Input: part model. Units: mm. Frame: model coordinates. Face numbers are marked on the shaded views. A direction names the side the tool comes from. Give positions to 0.01 mm unless a question says otherwise; leave off trailing zeros. Write each loop counter-clockwise with the first axis right and the second up, starting at its lowest first coordinate (ties: lowest second). Pieces come first, ordered by that corner, then holes. Notation, with made-up numbers: (77.25, -21.5) - (115.25, -21.5) arc R20 cw to (115.25, 1.5) - close; hole circle Ø8 at (5.25, 11). An arc over 180 degrees is marked (long way). Use a Markdown table: item, result. Add a question column.
1. Mould query, pull axis Y, two halves, no side actions, for the marked faces 1, 2, 3 and 4. Classes: released by +Y, released by -Y, zero draft, split by the parting line, or undercut.
2. Section query C-C, the plane z = -4. Return loops of the section in (x, y).
3. Pin query (flat end, axial travel): pin 1 (5 mm diameter, centred on x = -79, z = -7, fed in from +Y); pin 2 (4 mm diameter, centred on y = 70.5, z = -11.5, fed in from +X); pin 3 (5 mm diameter, centred on y = -74, z = -12.5, fed in from +X) (3 decimals); pin 4 (1.5 mm diameter, centred on x = -24.5, y = 76.5, fed in from +Z). Return the tip coordinate at first contact, or that it passes through.
4. Set-up query: the marked faces 5 and 6. Return all of +Z, -Z, +X, -X, +Y, -Y with unobstructed straight access to the full face (end or side cutting, diameter ignored); none if empty.
5. Section query B-B, the plane y = -5.5. Return loops of the section in (x, z) (3 decimals), plus the area to 3 significant figures.
6. Material intervals for probe 1 along Y at (x, z) = (50, 3.25); probe 2 along X at (y, z) = (-47.5, 0.25); probe 3 along Y at (x, z) = (-48.5, -2.5), sorted ascending.
7. Section query D-D, the plane y = 96. Return loops of the section in (x, z) (3 decimals).
```python
from build123d import *

# Parameters (mm, degrees)
F1_DEPTH = 15.875
F2_DEPTH = 9.525
F3_DEPTH = 6.35


with BuildPart() as f1:
    # F0 (on Top) → F1 (new body)
    with BuildSketch(Plane.XY):
        with BuildLine():
            ThreePointArc((-69.85, 109.5375), (-101.2808964237, 96.5183964237), (-114.3, 65.0875))
            Line((-114.3, 65.0875), (-114.3, -65.0875))
            ThreePointArc((-114.3, -65.0875), (-101.2808964237, -96.5183964237), (-69.85, -109.5375))
            Line((-69.85, -109.5375), (69.85, -109.5375))
            ThreePointArc((69.85, -109.5375), (101.2808964237, -96.5183964237), (114.3, -65.0875))
            Line((114.3, -65.0875), (114.3, 65.0875))
            ThreePointArc((114.3, 65.0875), (101.2808964237, 96.5183964237), (69.85, 109.5375))
            Line((69.85, 109.5375), (-69.85, 109.5375))
        make_face()
        with BuildLine():
            Line((-69.85, 103.187499407), (69.85, 103.187499407))
            ThreePointArc((69.85, 103.187499407), (96.7907679439, 92.0282679439), (107.949999407, 65.0875))
            Line((107.949999407, 65.0875), (107.949999407, -65.0875))
            ThreePointArc((107.949999407, -65.0875), (96.7907679439, -92.0282679439), (69.85, -103.187499407))
            Line((69.85, -103.187499407), (-69.85, -103.187499407))
            ThreePointArc((-69.85, -103.187499407), (-96.7907679439, -92.0282679439), (-107.949999407, -65.0875))
            Line((-107.949999407, -65.0875), (-107.949999407, 65.0875))
            ThreePointArc((-107.949999407, 65.0875), (-96.7907679439, 92.0282679439), (-69.85, 103.187499407))
        make_face(mode=Mode.SUBTRACT)
        with BuildLine():
            ThreePointArc((107.949999407, 65.0875), (96.7907679439, 92.0282679439), (69.85, 103.187499407))
            Line((69.85, 103.187499407), (-69.85, 103.187499407))
            ThreePointArc((-69.85, 103.187499407), (-96.7907679439, 92.0282679439), (-107.949999407, 65.0875))
            Line((-107.949999407, 65.0875), (-107.949999407, -65.0875))
            ThreePointArc((-107.949999407, -65.0875), (-96.7907679439, -92.0282679439), (-69.85, -103.187499407))
            Line((-69.85, -103.187499407), (69.85, -103.187499407))
            ThreePointArc((69.85, -103.187499407), (96.7907679439, -92.0282679439), (107.949999407, -65.0875))
            Line((107.949999407, -65.0875), (107.949999407, 65.0875))
        make_face()
        with BuildLine():
            Line((-107.187999407, -65.0875), (-107.187999407, 65.0875))
            ThreePointArc((-107.187999407, 65.0875), (-96.2519525766, 91.4894525766), (-69.85, 102.425499407))
            Line((-69.85, 102.425499407), (69.85, 102.425499407))
            ThreePointArc((69.85, 102.425499407), (96.2519525766, 91.4894525766), (107.187999407, 65.0875))
            Line((107.187999407, 65.0875), (107.187999407, -65.0875))
            ThreePointArc((107.187999407, -65.0875), (96.2519525766, -91.4894525766), (69.85, -102.425499407))
            Line((69.85, -102.425499407), (-69.85, -102.425499407))
            ThreePointArc((-69.85, -102.425499407), (-96.2519525766, -91.4894525766), (-107.187999407, -65.0875))
        make_face(mode=Mode.SUBTRACT)
        with BuildLine():
            ThreePointArc((-69.85, 102.425499407), (-96.2519525766, 91.4894525766), (-107.187999407, 65.0875))
            Line((-107.187999407, 65.0875), (-107.187999407, -65.0875))
            ThreePointArc((-107.187999407, -65.0875), (-96.2519525766, -91.4894525766), (-69.85, -102.425499407))
            Line((-69.85, -102.425499407), (69.85, -102.425499407))
            ThreePointArc((69.85, -102.425499407), (96.2519525766, -91.4894525766), (107.187999407, -65.0875))
            Line((107.187999407, -65.0875), (107.187999407, 65.0875))
            ThreePointArc((107.187999407, 65.0875), (96.2519525766, 91.4894525766), (69.85, 102.425499407))
            Line((69.85, 102.425499407), (-69.85, 102.425499407))
        make_face()
        with BuildLine():
            Line((-89.662, -65.0875), (-89.662, 65.0875))
            ThreePointArc((-89.662, 65.0875), (-83.8591995489, 79.0966995489), (-69.85, 84.8995))
            Line((-69.85, 84.8995), (69.85, 84.8995))
            ThreePointArc((69.85, 84.8995), (83.8591995489, 79.0966995489), (89.662, 65.0875))
            Line((89.662, 65.0875), (89.662, -65.0875))
            ThreePointArc((89.662, -65.0875), (83.8591995489, -79.0966995489), (69.85, -84.8995))
            Line((69.85, -84.8995), (-69.85, -84.8995))
            ThreePointArc((-69.85, -84.8995), (-83.8591995489, -79.0966995489), (-89.662, -65.0875))
        make_face(mode=Mode.SUBTRACT)
        with BuildLine():
            ThreePointArc((-69.85, 84.8995), (-83.8591995489, 79.0966995489), (-89.662, 65.0875))
            Line((-89.662, 65.0875), (-89.662, -65.0875))
            ThreePointArc((-89.662, -65.0875), (-83.8591995489, -79.0966995489), (-69.85, -84.8995))
            Line((-69.85, -84.8995), (69.85, -84.8995))
            ThreePointArc((69.85, -84.8995), (83.8591995489, -79.0966995489), (89.662, -65.0875))
            Line((89.662, -65.0875), (89.662, 65.0875))
            ThreePointArc((89.662, 65.0875), (83.8591995489, 79.0966995489), (69.85, 84.8995))
            Line((69.85, 84.8995), (-69.85, 84.8995))
        make_face()
        with BuildLine():
            ThreePointArc((-88.9, 65.0875), (-83.3203841816, 78.5578841816), (-69.85, 84.1375))
            Line((-69.85, 84.1375), (69.85, 84.1375))
            ThreePointArc((69.85, 84.1375), (83.3203841816, 78.5578841816), (88.9, 65.0875))
            Line((88.9, 65.0875), (88.9, -65.0875))
            ThreePointArc((88.9, -65.0875), (83.3203841816, -78.5578841816), (69.85, -84.1375))
            Line((69.85, -84.1375), (-69.85, -84.1375))
            ThreePointArc((-69.85, -84.1375), (-83.3203841816, -78.5578841816), (-88.9, -65.0875))
            Line((-88.9, -65.0875), (-88.9, 65.0875))
        make_face(mode=Mode.SUBTRACT)
        with BuildLine():
            Line((69.85, 84.1375), (-69.85, 84.1375))
            ThreePointArc((-69.85, 84.1375), (-83.3203841816, 78.5578841816), (-88.9, 65.0875))
            Line((-88.9, 65.0875), (-88.9, -65.0875))
            ThreePointArc((-88.9, -65.0875), (-83.3203841816, -78.5578841816), (-69.85, -84.1375))
            Line((-69.85, -84.1375), (69.85, -84.1375))
            ThreePointArc((69.85, -84.1375), (83.3203841816, -78.5578841816), (88.9, -65.0875))
            Line((88.9, -65.0875), (88.9, 65.0875))
            ThreePointArc((88.9, 65.0875), (83.3203841816, 78.5578841816), (69.85, 84.1375))
        make_face()
        with BuildLine():
            Line((-69.85, 77.7875), (69.85, 77.7875))
            ThreePointArc((69.85, 77.7875), (78.8302561211, 74.0677561211), (82.55, 65.0875))
            Line((82.55, 65.0875), (82.55, -65.0875))
            ThreePointArc((82.55, -65.0875), (78.8302561211, -74.0677561211), (69.85, -77.7875))
            Line((69.85, -77.7875), (-69.85, -77.7875))
            ThreePointArc((-69.85, -77.7875), (-78.8302561211, -74.0677561211), (-82.55, -65.0875))
            Line((-82.55, -65.0875), (-82.55, 65.0875))
            ThreePointArc((-82.55, 65.0875), (-78.8302561211, 74.0677561211), (-69.85, 77.7875))
        make_face(mode=Mode.SUBTRACT)
    extrude(amount=-F1_DEPTH)

    # F0 (on Top) → F2 (cut)
    with BuildSketch(Plane.XY):
        with BuildLine():
            ThreePointArc((107.949999407, 65.0875), (96.7907679439, 92.0282679439), (69.85, 103.187499407))
            Line((69.85, 103.187499407), (-69.85, 103.187499407))
            ThreePointArc((-69.85, 103.187499407), (-96.7907679439, 92.0282679439), (-107.949999407, 65.0875))
            Line((-107.949999407, 65.0875), (-107.949999407, -65.0875))
            ThreePointArc((-107.949999407, -65.0875), (-96.7907679439, -92.0282679439), (-69.85, -103.187499407))
            Line((-69.85, -103.187499407), (69.85, -103.187499407))
            ThreePointArc((69.85, -103.187499407), (96.7907679439, -92.0282679439), (107.949999407, -65.0875))
            Line((107.949999407, -65.0875), (107.949999407, 65.0875))
        make_face()
        with BuildLine():
            Line((-107.187999407, -65.0875), (-107.187999407, 65.0875))
            ThreePointArc((-107.187999407, 65.0875), (-96.2519525766, 91.4894525766), (-69.85, 102.425499407))
            Line((-69.85, 102.425499407), (69.85, 102.425499407))
            ThreePointArc((69.85, 102.425499407), (96.2519525766, 91.4894525766), (107.187999407, 65.0875))
            Line((107.187999407, 65.0875), (107.187999407, -65.0875))
            ThreePointArc((107.187999407, -65.0875), (96.2519525766, -91.4894525766), (69.85, -102.425499407))
            Line((69.85, -102.425499407), (-69.85, -102.425499407))
            ThreePointArc((-69.85, -102.425499407), (-96.2519525766, -91.4894525766), (-107.187999407, -65.0875))
        make_face(mode=Mode.SUBTRACT)
        with BuildLine():
            ThreePointArc((-69.85, 102.425499407), (-96.2519525766, 91.4894525766), (-107.187999407, 65.0875))
            Line((-107.187999407, 65.0875), (-107.187999407, -65.0875))
            ThreePointArc((-107.187999407, -65.0875), (-96.2519525766, -91.4894525766), (-69.85, -102.425499407))
            Line((-69.85, -102.425499407), (69.85, -102.425499407))
            ThreePointArc((69.85, -102.425499407), (96.2519525766, -91.4894525766), (107.187999407, -65.0875))
            Line((107.187999407, -65.0875), (107.187999407, 65.0875))
            ThreePointArc((107.187999407, 65.0875), (96.2519525766, 91.4894525766), (69.85, 102.425499407))
            Line((69.85, 102.425499407), (-69.85, 102.425499407))
        make_face()
        with BuildLine():
            Line((-89.662, -65.0875), (-89.662, 65.0875))
            ThreePointArc((-89.662, 65.0875), (-83.8591995489, 79.0966995489), (-69.85, 84.8995))
            Line((-69.85, 84.8995), (69.85, 84.8995))
            ThreePointArc((69.85, 84.8995), (83.8591995489, 79.0966995489), (89.662, 65.0875))
            Line((89.662, 65.0875), (89.662, -65.0875))
            ThreePointArc((89.662, -65.0875), (83.8591995489, -79.0966995489), (69.85, -84.8995))
            Line((69.85, -84.8995), (-69.85, -84.8995))
            ThreePointArc((-69.85, -84.8995), (-83.8591995489, -79.0966995489), (-89.662, -65.0875))
        make_face(mode=Mode.SUBTRACT)
    extrude(amount=F2_DEPTH, mode=Mode.SUBTRACT)

    # F0 (on Top) → F3 (join)
    with BuildSketch(Plane.XY):
        with BuildLine():
            ThreePointArc((-69.85, 109.5375), (-101.2808964237, 96.5183964237), (-114.3, 65.0875))
            Line((-114.3, 65.0875), (-114.3, -65.0875))
            ThreePointArc((-114.3, -65.0875), (-101.2808964237, -96.5183964237), (-69.85, -109.5375))
            Line((-69.85, -109.5375), (69.85, -109.5375))
            ThreePointArc((69.85, -109.5375), (101.2808964237, -96.5183964237), (114.3, -65.0875))
            Line((114.3, -65.0875), (114.3, 65.0875))
            ThreePointArc((114.3, 65.0875), (101.2808964237, 96.5183964237), (69.85, 109.5375))
            Line((69.85, 109.5375), (-69.85, 109.5375))
        make_face()
        with BuildLine():
            Line((-69.85, 103.187499407), (69.85, 103.187499407))
            ThreePointArc((69.85, 103.187499407), (96.7907679439, 92.0282679439), (107.949999407, 65.0875))
            Line((107.949999407, 65.0875), (107.949999407, -65.0875))
            ThreePointArc((107.949999407, -65.0875), (96.7907679439, -92.0282679439), (69.85, -103.187499407))
            Line((69.85, -103.187499407), (-69.85, -103.187499407))
            ThreePointArc((-69.85, -103.187499407), (-96.7907679439, -92.0282679439), (-107.949999407, -65.0875))
            Line((-107.949999407, -65.0875), (-107.949999407, 65.0875))
            ThreePointArc((-107.949999407, 65.0875), (-96.7907679439, 92.0282679439), (-69.85, 103.187499407))
        make_face(mode=Mode.SUBTRACT)
        with BuildLine():
            Line((69.85, 84.1375), (-69.85, 84.1375))
            ThreePointArc((-69.85, 84.1375), (-83.3203841816, 78.5578841816), (-88.9, 65.0875))
            Line((-88.9, 65.0875), (-88.9, -65.0875))
            ThreePointArc((-88.9, -65.0875), (-83.3203841816, -78.5578841816), (-69.85, -84.1375))
            Line((-69.85, -84.1375), (69.85, -84.1375))
            ThreePointArc((69.85, -84.1375), (83.3203841816, -78.5578841816), (88.9, -65.0875))
            Line((88.9, -65.0875), (88.9, 65.0875))
            ThreePointArc((88.9, 65.0875), (83.3203841816, 78.5578841816), (69.85, 84.1375))
        make_face()
        with BuildLine():
            Line((-69.85, 77.7875), (69.85, 77.7875))
            ThreePointArc((69.85, 77.7875), (78.8302561211, 74.0677561211), (82.55, 65.0875))
            Line((82.55, 65.0875), (82.55, -65.0875))
            ThreePointArc((82.55, -65.0875), (78.8302561211, -74.0677561211), (69.85, -77.7875))
            Line((69.85, -77.7875), (-69.85, -77.7875))
            ThreePointArc((-69.85, -77.7875), (-78.8302561211, -74.0677561211), (-82.55, -65.0875))
            Line((-82.55, -65.0875), (-82.55, 65.0875))
            ThreePointArc((-82.55, 65.0875), (-78.8302561211, 74.0677561211), (-69.85, 77.7875))
        make_face(mode=Mode.SUBTRACT)
    extrude(amount=F3_DEPTH)


solid = f1.part
```
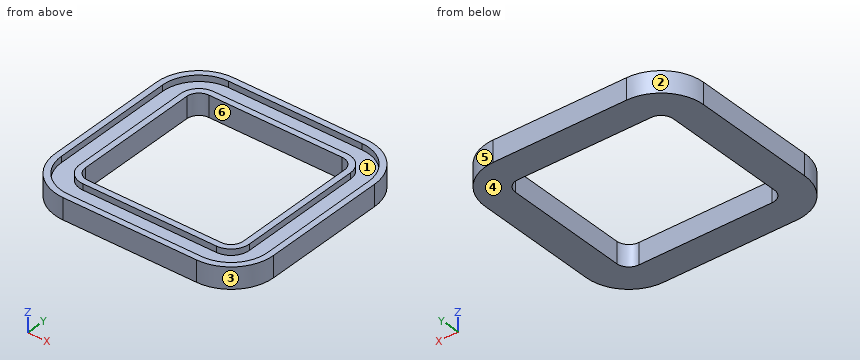
Result sheet:
| question | item | result |
|---|---|---|
| 1 | face 1 | undercut |
| 1 | face 2 | released by +Y |
| 1 | face 3 | released by -Y |
| 1 | face 4 | zero draft |
| 2 | outline | (-114.3, -65.09) arc R44.45 ccw to (-69.85, -109.54) - (69.85, -109.54) arc R44.45 ccw to (114.3, -65.09) - (114.3, 65.09) arc R44.45 ccw to (69.85, 109.54) - (-69.85, 109.54) arc R44.45 ccw to (-114.3, 65.09) - close; hole (-82.55, -65.09) arc R12.7 ccw to (-69.85, -77.79) - (69.85, -77.79) arc R12.7 ccw to (82.55, -65.09) - (82.55, 65.09) arc R12.7 ccw to (69.85, 77.79) - (-69.85, 77.79) arc R12.7 ccw to (-82.55, 65.09) - close |
| 3 | pin 1 | stops at y = 109.04 |
| 3 | pin 2 | stops at x = 114.17 |
| 3 | pin 3 | stops at x = 113.835 |
| 3 | pin 4 | passes through |
| 4 | face 5 | +Z, -Z, +X, +Y |
| 4 | face 6 | +Z, -Z |
| 5 | outline | (-114.3, -15.875) - (-82.55, -15.875) - (-82.55, 6.35) - (-88.9, 6.35) - (-88.9, 0) - (-107.95, 0) - (-107.95, 6.35) - (-114.3, 6.35) - close; (82.55, -15.875) - (114.3, -15.875) - (114.3, 6.35) - (107.95, 6.35) - (107.95, 0) - (88.9, 0) - (88.9, 6.35) - (82.55, 6.35) - close |
| 5 | area | 1,170 mm² |
| 6 | probe 1 | y = -109.54 to -103.19, -84.14 to -77.79, 77.79 to 84.14, 103.19 to 109.54 |
| 6 | probe 2 | x = -114.3 to -107.95, -88.9 to -82.55, 82.55 to 88.9, 107.95 to 114.3 |
| 6 | probe 3 | y = -109.54 to -77.79, 77.79 to 109.54 |
| 7 | outline | (-101.791, -15.875) - (101.791, -15.875) - (101.791, 6.35) - (92.122, 6.35) - (92.122, 0) - (-92.122, 0) - (-92.122, 6.35) - (-101.791, 6.35) - close |
